Here's how the part is built. I have some questions about the finished solid (model axes, mm). Face numbers are marked on the shaded views. A direction names the side the tool comes from. Round coordinates to 2 decimals unless told otherwise and drop trailing zeros. Loops run counter-clockwise (first coordinate to the right, second up) from the corner with the lowest first, then second, coordinate; pieces in that order, holes last. Notation, with made-up numbers: M -8,62 L 27,62 A29 ccw 27,92 Z; hole C 86.5,66 d5. An arc over 180 degrees is marked long. Answer as a JSON object with one key per item and string values.
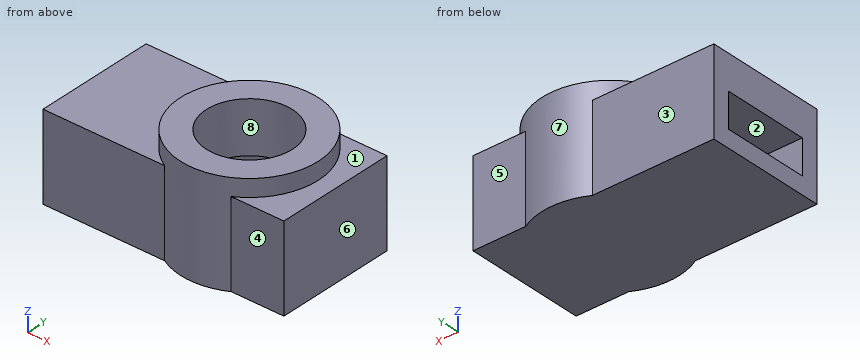
from build123d import *

# Parameters (mm, degrees)
SKETCH1_W                = 4
SKETCH1_H                = 7
SKETCH1_W_2              = 2
SKETCH1_H_2              = 5
SKETCH1_W_3              = 1
BOSS_EXTRUDE1_DEPTH      = 14
SKETCH2_R                = 2.5
CUT_EXTRUDE1_DEPTH       = 14
BOSS_EXTRUDE3_DEPTH      = 1
BOSS_EXTRUDE3_DEPTH_BACK = 5
SKETCH3_R                = 4
SKETCH3_R_2              = 2.5
SKETCH4_W                = 2
SKETCH4_H                = 5
CUT_EXTRUDE2_DEPTH       = 16.099668871
SKETCH6_W                = 5.975626827
SKETCH6_H                = 5.438491831
BOSS_EXTRUDE4_DEPTH      = 0.5
SKETCH7_W                = 2
SKETCH7_H                = 5
BOSS_EXTRUDE5_DEPTH      = 2


with BuildPart() as part:
    # Sketch1 → Boss-Extrude1 (new body)
    # profile 1 of 2: a face of its own
    with BuildSketch(Plane(origin=(0, 0, 0), x_dir=(0, 0, -1), z_dir=(1, 0, 0))):
        Rectangle(SKETCH1_W, SKETCH1_H)
        Rectangle(SKETCH1_W_2, SKETCH1_H_2, mode=Mode.SUBTRACT)
    # profile 2 of 2: a face of its own
    with BuildSketch(Plane(origin=(0, 0, 0), x_dir=(0, 0, -1), z_dir=(1, 0, 0))):
        with Locations((-2.5, 0)):
            Rectangle(SKETCH1_W_3, SKETCH1_H)
    extrude(amount=BOSS_EXTRUDE1_DEPTH)

    # Sketch2 → Cut-Extrude1 (cut)
    with BuildSketch(Plane.XY.offset(3)):
        with Locations((9, 0)):
            Circle(SKETCH2_R)
    extrude(amount=-CUT_EXTRUDE1_DEPTH, mode=Mode.SUBTRACT)

    # Sketch3 → Boss-Extrude3 (add, two sides: drawn at the far end of the back side and taken through both)
    with BuildSketch(Plane.XY.offset(3).offset(-BOSS_EXTRUDE3_DEPTH_BACK)):
        with Locations((9, 0)):
            Circle(SKETCH3_R)
        with Locations((9, 0)):
            Circle(SKETCH3_R_2, mode=Mode.SUBTRACT)
    extrude(amount=BOSS_EXTRUDE3_DEPTH + BOSS_EXTRUDE3_DEPTH_BACK)

    # Sketch4 → Cut-Extrude2 (cut, through all)
    with BuildSketch(Plane(origin=(14, 0, 0), x_dir=(0, 0, -1), z_dir=(1, 0, 0))):
        Rectangle(SKETCH4_W, SKETCH4_H)
    extrude(amount=-CUT_EXTRUDE2_DEPTH, mode=Mode.SUBTRACT)

    # Sketch6 → Boss-Extrude4 (add)
    with BuildSketch(Plane(origin=(0, 0, -2), x_dir=(-1, 0, 0), z_dir=(0, 0, -1))):
        with Locations((-9.038624366, 0.008392735)):
            Rectangle(SKETCH6_W, SKETCH6_H)
    extrude(amount=-BOSS_EXTRUDE4_DEPTH)

    # Sketch7 → Boss-Extrude5 (add)
    with BuildSketch(Plane(origin=(14, 0, 0), x_dir=(0, 0, -1), z_dir=(1, 0, 0))):
        Rectangle(SKETCH7_W, SKETCH7_H)
    extrude(amount=-BOSS_EXTRUDE5_DEPTH)


solid = part.part
Item 1: I want a section at B-B, the plane x = 2.5. Please give me the cut outline in (y, z), then the cut area to 3 significant figures.
Resolved:
{"outline": "M -3.5,-2 L 3.5,-2 L 3.5,3 L -3.5,3 Z; hole M -2.5,-1 L 2.5,-1 L 2.5,1 L -2.5,1 Z", "area": "25.0 mm²"}
Item 2: I want a section at A-A, the plane y = 0. Please give me the cut outline in (x, z), then the cut area to 3 significant figures.
Resolved:
{"outline": "M 0,-2 L 14,-2 L 14,3 L 13,3 L 13,4 L 11.5,4 L 11.5,1 L 12,1 L 12,-1 L 11.5,-1 L 11.5,-1.5 L 6.5,-1.5 L 6.5,-1 L 0,-1 Z; M 0,1 L 6.5,1 L 6.5,4 L 5,4 L 5,3 L 0,3 Z", "area": "36.5 mm²"}
Item 3: I'm going to push flat-ended pins straight in: pin 1 Ø2 at (x, z) = (4, 0.5) entering from -Y; pin 2 Ø1.5 at (x, y) = (8, 0.5) entering from +Z; pin 3 Ø2.5 at (x, z) = (12, 1.5) entering from +Y. Where does each tip first touch, or does it pass through?
Resolved:
{"pin 1": "y = -3.5", "pin 2": "z = -1.5", "pin 3": "y = 3.6"}
Item 4: Please list where these lines run through material, in increasing order: probe 1 along X at (y, z) = (0, 2.9); probe 2 along Y at (x, z) = (3, -0.4); probe 3 along Z at (x, y) = (6, 1). Write a range as from..to.
Resolved:
{"probe 1": "0..6.5, 11.5..14", "probe 2": "-3.5..-2.5, 2.5..3.5", "probe 3": "-2..-1, 1..4"}
Item 5: I want a section at D-D, the plane z = 0.4. Please give me the cut outline in (x, y).
Resolved:
{"outline": "M 0,-3.5 L 7.06,-3.5 A4 ccw 10.94,-3.5 L 14,-3.5 L 14,3.5 L 10.94,3.5 A4 ccw 7.06,3.5 L 0,3.5 L 0,2.5 L 12,2.5 L 12,-2.5 L 0,-2.5 Z"}
Item 6: On a 3-axis mill with a long thin cutter (end or side, diameter ignored), from which of +Z, -Z, +X, -X, +Y, -Y can I reach the whole of each face in a straight line? I mean the marked faces 1, 2, 3 and 4. Say none if no direction works.
Resolved:
{"face 1": "+Z, +X", "face 2": "-X", "face 3": "+Z, -Z, -X, +Y", "face 4": "+Z, -Z, +X, -Y"}
Item 7: I want a section at C-C, the plane z = 2.85. Please give me the cut outline in (x, y), then the cut area to 3 significant figures.
Resolved:
{"outline": "M 0,-3.5 L 7.06,-3.5 A4 ccw 10.94,-3.5 L 14,-3.5 L 14,3.5 L 10.94,3.5 A4 ccw 7.06,3.5 L 0,3.5 Z; hole C 9,0 d5", "area": "81.0 mm²"}
Item 8: If we mould it in two halves opening along X, with no side actions, what happens to the marked faces 5, 6, 7 and 8? For each: pulls with the +X half, pulls with the -X half, needs draft (parallel to the pull), parting line crosses it, or undercut.
Resolved:
{"face 5": "needs draft", "face 6": "pulls with the +X half", "face 7": "parting line crosses it", "face 8": "undercut"}
